Input: part model. Units: mm. Frame: model coordinates. A direction names the side the tool comes from. Round coordinates to 2 decimals unless told otherwise and drop trailing zeros. Write each loop counter-clockwise with the first axis right and the second up, starting at its lowest first coordinate (ties: lowest second). Pieces come first, ordered by that corner, then holes. Notation, with made-up numbers: (82.25, 55.5) -> (140.25, 55.5) arc R33 cw to (140.25, 90.5) -> close; hole circle Ø2 at (12.25, 83). An arc over 180 degrees is marked (long way). Use CSV: the item, a comma, the result in double quotes.
```python
from build123d import *

# Parameters (mm, degrees)
SKETCH2_W           = 30
SKETCH2_H           = 30
SKETCH2_R           = 12.55
BOSS_EXTRUDE1_DEPTH = 5
SKETCH4_W           = 30
SKETCH4_H           = 30
BOSS_EXTRUDE2_DEPTH = 1


with BuildPart() as part:
    # Sketch2 → Boss-Extrude1 (new body)
    with BuildSketch(Plane.XY):
        Rectangle(SKETCH2_W, SKETCH2_H)
        Circle(SKETCH2_R, mode=Mode.SUBTRACT)
    extrude(amount=-BOSS_EXTRUDE1_DEPTH)

    # Sketch4 → Boss-Extrude2 (add)
    with BuildSketch(Plane.XY):
        Rectangle(SKETCH4_W, SKETCH4_H)
    extrude(amount=BOSS_EXTRUDE2_DEPTH)


solid = part.part
```
Item 1: Section query A-A on x = 0. Return the cut outline in (y, z).
Worked answers:
outline,"(-15, -5) -> (-12.55, -5) -> (-12.55, 0) -> (12.55, 0) -> (12.55, -5) -> (15, -5) -> (15, 1) -> (-15, 1) -> close"
Item 2: Pull-direction query (X, two-part tool) for faces 3 (the face through (15, 0, -2)), 4 (the face through (11.59, -4.81, -2.46)), 5 (the face through (0, 0, 1)), 6 (the face through (-15, 0, -2)); classes: +X half, -X half, draft (parallel to the pull), parting line (faces both ways), or undercut.
Worked answers:
face 3,"+X half"
face 4,"undercut"
face 5,"draft"
face 6,"-X half"
Item 3: First-contact query: pin 1 Ø4 at (x, y) = (3, -10.5) entering from -Z; pin 2 Ø3 at (x, y) = (-7, 6.5) entering from -Z. Flat tips, straight axial feed; report the tip coordinate or a pass-through.
Worked answers:
pin 1,"stops at z = -5"
pin 2,"stops at z = 0"
Item 4: Line query: line 1 (Y direction, x = 0, z = -3.4); line 2 (Z direction, x = -6.5, y = 3.5); line 3 (X direction, y = 4.75, z = -3.45). Output: solid intervals per line, ascending.
Worked answers:
line 1,"y = -15 to -12.55, 12.55 to 15"
line 2,"z = 0 to 1"
line 3,"x = -15 to -11.62, 11.62 to 15"
Item 5: Set-up query: faces 1 (the face through (0, 15, -2)), 2 (the face through (0, 0, 0)). Return all of +Z, -Z, +X, -X, +Y, -Y with unobstructed straight access to the full face (end or side cutting, diameter ignored); none if empty.
Worked answers:
face 1,"+Z, -Z, +X, -X, +Y"
face 2,"-Z"
Item 6: Section query C-C on z = -2. Return the cut outline in (x, y), plus the area to 3 significant figures.
Worked answers:
outline,"(-15, -15) -> (15, -15) -> (15, 15) -> (-15, 15) -> close; hole circle Ø25.1 at (0, 0)"
area,"405 mm²"
